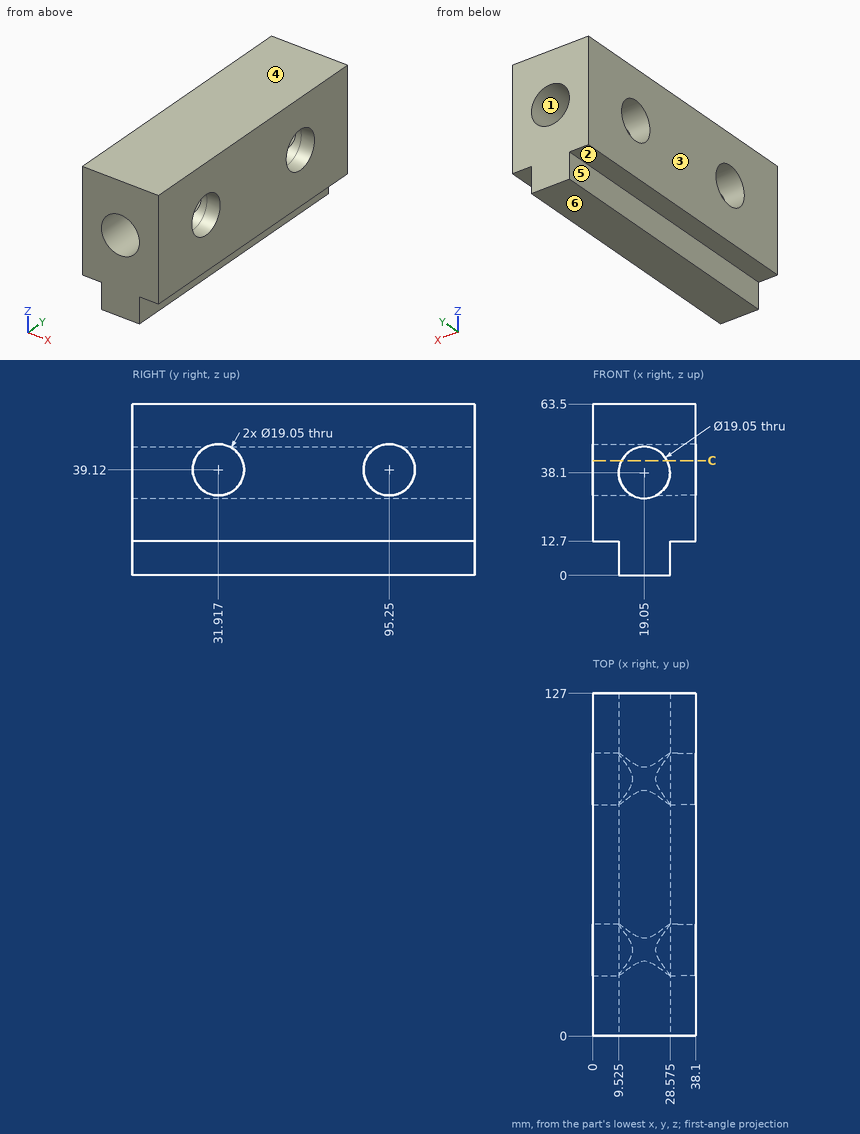
Design review of the part shown in the three views and the two pictorial views. Dimensions are in mm from the part's minimum x, y and z. A direction names the side the tool comes from. Give positions to 0.01 mm unless a question says otherwise; leave off trailing zeros. Loops run counter-clockwise (first coordinate to the right, second up) from the corner with the lowest first, then second, coordinate; pieces in that order, holes last. Notation, with made-up numbers: (-14.75, 30.5) -> (41.25, 30.5) arc R19 ccw to (41.25, 45.5) -> close; hole circle Ø4 at (9.25, -39.5). An arc over 180 degrees is marked (long way). Write each question's results on one line, items separated by ' | '.
Q1. Take a section at C-C, the plane z = 42.5. Write out the cut boundary in (x, y) (1 decimal), plus the area to 3 significant figures.
Reply:
outline: (0, 0) -> (10.6, 0) -> (10.6, 23) -> (0, 23) -> close; (0, 40.8) -> (10.6, 40.8) -> (10.6, 86.3) -> (0, 86.3) -> close; (0, 104.2) -> (10.6, 104.2) -> (10.6, 127) -> (0, 127) -> close; (27.5, 0) -> (38.1, 0) -> (38.1, 23) -> (27.5, 23) -> close; (27.5, 40.8) -> (38.1, 40.8) -> (38.1, 86.3) -> (27.5, 86.3) -> close; (27.5, 104.2) -> (38.1, 104.2) -> (38.1, 127) -> (27.5, 127) -> close | area: 1,940 mm²
Q2. Machinability: for the marked faces 5 and 6, which of the approach directions +Z, -Z, +X, -X, +Y, -Y give a long, thin tool a straight path to every point of the face, cutting with its end or side? Answer none if there is none.
Reply:
face 5: -Z, -X, +Y, -Y | face 6: -Z, +X, -X, +Y, -Y
Q3. Wall thickness on L1, parallel to Y at x = 4, z = 39 (1 decimal); L2, parallel to X at y = 107, z = 38.5; L3, parallel to Y at x = 2, z = 44 (1 decimal): over which ranges is each line inside the solid? List them lowest first.
Reply:
L1: y = 0 to 22.4, 41.4 to 85.7, 104.8 to 127 | L2: x = 0 to 9.53, 28.57 to 38.1 | L3: y = 0 to 23.7, 40.1 to 87.1, 103.4 to 127
Q4. For pin 1 Ø4 at (y, z) = (62, 4.5) entering from +X (3 decimals); pin 2 Ø10.5 at (x, y) = (34, 64.5) entering from -Z; pin 3 Ø6.5 at (y, z) = (66, 8) entering from -X (3 decimals), all flat-tipped, find the tip position at first contact; note any pin that passes through.
Reply:
pin 1: stops at x = 28.575 | pin 2: stops at z = 12.7 | pin 3: stops at x = 9.525
Q5. The part is to be moulded in two halves that separate along Z. For the marked faces 1, 2, 3 and 4, say which applies: +Z half, -Z half, draft (parallel to the pull), parting line (faces both ways), or undercut.
Reply:
face 1: undercut | face 2: -Z half | face 3: draft | face 4: +Z half
